Here's how the part is built. I have some questions about the finished solid (model axes, mm). A direction names the side the tool comes from. Coordinates: 2 decimals unless noted, no trailing zeros. Order: outer loops, then holes, each group sorted by start corner. A loop starts at its lowest first (then second) coordinate and runs counter-clockwise, first axis right, second up. Notation, with made-up numbers: (76.25, 55) - (94.25, 55) arc R31 cw to (94.25, 89) - close; hole circle Ø5 at (-29, 45.25). An arc over 180 degrees is marked (long way). Answer as CSV lines item,"result". Start each with the question number.
Q1. For faces 5 (the face through (-12, 0, -1.5)), 6 (the face through (-12, 0, 1.5)), 7 (the face through (-0.08, -0.62, 8.93)), which set-ups out of +Z, -Z, +X, -X, +Y, -Y let a thin tool reach every point of the face, with its end or its side?
Q2. Thinking about a two-plate mould opening in Z: for faces 1 (the face through (12, 0, 1.5)), 2 (the face through (-5, 1, 8)), 3 (the face through (12, 0, -1.5)), 4 (the face through (13.196, -0.014, -0.065)), which applies, released by +Z, released by -Z, zero draft, split by the parting line, or undercut?
Q3. I need wall thicknesses on line 1 (X direction, y = 0.65, z = 2.5); line 2 (X direction, y = -0.5, z = -3.25); line 3 (Z direction, x = 11.5, y = 0.8). Which ranges of each line are inside material? Lowest first, please.
Q4. Suppose I cut it at C-C (x = -10.25). Please give me the cut outline in (y, z).
Q5. Suppose I cut it at A-A (x = 12.7). Please give me the cut outline in (y, z).
Q6. Suppose I cut it at B-B (y = -0.35). Count the separate pieces of the cut face and the enclosed holes in it, then the cut area to 3 significant figures.
Q7. For pin 1 Ø1 at (x, y) = (-1, 0) entering from -Z; pin 2 Ø8 at (x, z) = (3.5, 3) entering from +Y; pin 3 Ø1 at (x, y) = (-8, -0.5) entering from -Z; pin 4 Ø8 at (x, z) = (-7.5, 1.5) entering from +Y, each with a flat end and sliding along its axis, tell me the tip position at first contact or that it passes through.
from build123d import *

# Parameters (mm, degrees)
SKETCH1_R           = 0.5
BOSS_EXTRUDE1_DEPTH = 1
CUT_EXTRUDE1_START  = -15
CUT_EXTRUDE1_DEPTH  = 30


with BuildPart() as part:
    # Sketch1 → Boss-Extrude1 (new, symmetric)
    # profile 1 of 14: a face of its own
    with BuildSketch(Plane(origin=(0, 0, 0), x_dir=(1, 0, 0), z_dir=(0, 1, 0))):
        with BuildLine():
            Line((-15, -1.5), (-9.886859967, -1.5))
            ThreePointArc((-9.886859967, -1.5), (-10, 0), (-9.886859967, 1.5))
            Line((-9.886859967, 1.5), (-15, 1.5))
            Line((-15, 1.5), (-15, -1.5))
        make_face()
        with Locations(Location((-12.7, 0, 0), (0, 0, 270))):
            Circle(SKETCH1_R, mode=Mode.SUBTRACT)
    # profile 2 of 14: a face of its own
    with BuildSketch(Plane(origin=(0, 0, 0), x_dir=(1, 0, 0), z_dir=(0, 1, 0))):
        with BuildLine():
            ThreePointArc((-9.886859967, 1.5), (-10, 0), (-9.886859967, -1.5))
            Line((-9.886859967, -1.5), (-8.874119675, -1.5))
            ThreePointArc((-8.874119675, -1.5), (-9, 0), (-8.874119675, 1.5))
            Line((-8.874119675, 1.5), (-9.886859967, 1.5))
        make_face()
    # profile 3 of 14: a face of its own
    with BuildSketch(Plane(origin=(0, 0, 0), x_dir=(1, 0, 0), z_dir=(0, 1, 0))):
        with BuildLine():
            Line((8.874119675, -1.5), (9.886859967, -1.5))
            ThreePointArc((9.886859967, -1.5), (9.971674876, -0.752130419), (10, 0))
            ThreePointArc((10, 0), (9.971674876, 0.752130419), (9.886859967, 1.5))
            Line((9.886859967, 1.5), (8.874119675, 1.5))
            ThreePointArc((8.874119675, 1.5), (8.968474705, 0.752636343), (9, 0))
            ThreePointArc((9, 0), (8.968474705, -0.752636343), (8.874119675, -1.5))
        make_face()
    # profile 4 of 14: a face of its own
    with BuildSketch(Plane(origin=(0, 0, 0), x_dir=(1, 0, 0), z_dir=(0, 1, 0))):
        with BuildLine():
            ThreePointArc((-9.886859967, -1.5), (-6.519202405, -7.582875444), (0, -10))
            Line((0, -10), (0, -9))
            ThreePointArc((0, -9), (-5.809475019, -6.873863542), (-8.874119675, -1.5))
            Line((-8.874119675, -1.5), (-9.886859967, -1.5))
        make_face()
    # profile 5 of 14: a face of its own
    with BuildSketch(Plane(origin=(0, 0, 0), x_dir=(1, 0, 0), z_dir=(0, 1, 0))):
        with BuildLine():
            Line((0, -9), (0, -10))
            ThreePointArc((0, -10), (6.519202405, -7.582875444), (9.886859967, -1.5))
            Line((9.886859967, -1.5), (8.874119675, -1.5))
            ThreePointArc((8.874119675, -1.5), (5.809475019, -6.873863542), (0, -9))
        make_face()
    # profile 6 of 14: a face of its own
    with BuildSketch(Plane(origin=(0, 0, 0), x_dir=(1, 0, 0), z_dir=(0, 1, 0))):
        with BuildLine():
            ThreePointArc((0, 10), (-6.519202405, 7.582875444), (-9.886859967, 1.5))
            Line((-9.886859967, 1.5), (-8.874119675, 1.5))
            ThreePointArc((-8.874119675, 1.5), (-5.809475019, 6.873863542), (0, 9))
            Line((0, 9), (0, 10))
        make_face()
    # profile 7 of 14: a face of its own
    with BuildSketch(Plane(origin=(0, 0, 0), x_dir=(1, 0, 0), z_dir=(0, 1, 0))):
        with BuildLine():
            ThreePointArc((9.886859967, 1.5), (6.519202405, 7.582875444), (0, 10))
            Line((0, 10), (0, 9))
            ThreePointArc((0, 9), (5.809475019, 6.873863542), (8.874119675, 1.5))
            Line((8.874119675, 1.5), (9.886859967, 1.5))
        make_face()
    # profile 8 of 14: a face of its own
    with BuildSketch(Plane(origin=(0, 0, 0), x_dir=(1, 0, 0), z_dir=(0, 1, 0))):
        with BuildLine():
            ThreePointArc((-9.886859967, -1.5), (-6.519202405, -7.582875444), (0, -10))
            Line((0, -10), (0, -9))
            ThreePointArc((0, -9), (-5.809475019, -6.873863542), (-8.874119675, -1.5))
            Line((-8.874119675, -1.5), (-9.886859967, -1.5))
        make_face()
    # profile 9 of 14: a face of its own
    with BuildSketch(Plane(origin=(0, 0, 0), x_dir=(1, 0, 0), z_dir=(0, 1, 0))):
        with BuildLine():
            Line((0, -9), (0, -10))
            ThreePointArc((0, -10), (6.519202405, -7.582875444), (9.886859967, -1.5))
            Line((9.886859967, -1.5), (8.874119675, -1.5))
            ThreePointArc((8.874119675, -1.5), (5.809475019, -6.873863542), (0, -9))
        make_face()
    # profile 10 of 14: a face of its own
    with BuildSketch(Plane(origin=(0, 0, 0), x_dir=(1, 0, 0), z_dir=(0, 1, 0))):
        with BuildLine():
            ThreePointArc((0, 10), (-6.519202405, 7.582875444), (-9.886859967, 1.5))
            Line((-9.886859967, 1.5), (-8.874119675, 1.5))
            ThreePointArc((-8.874119675, 1.5), (-5.809475019, 6.873863542), (0, 9))
            Line((0, 9), (0, 10))
        make_face()
    # profile 11 of 14: a face of its own
    with BuildSketch(Plane(origin=(0, 0, 0), x_dir=(1, 0, 0), z_dir=(0, 1, 0))):
        with BuildLine():
            ThreePointArc((9.886859967, 1.5), (6.519202405, 7.582875444), (0, 10))
            Line((0, 10), (0, 9))
            ThreePointArc((0, 9), (5.809475019, 6.873863542), (8.874119675, 1.5))
            Line((8.874119675, 1.5), (9.886859967, 1.5))
        make_face()
    # profile 12 of 14: a face of its own
    with BuildSketch(Plane(origin=(0, 0, 0), x_dir=(1, 0, 0), z_dir=(0, 1, 0))):
        with BuildLine():
            ThreePointArc((10, 0), (9.971674876, -0.752130419), (9.886859967, -1.5))
            Line((9.886859967, -1.5), (15, -1.5))
            Line((15, -1.5), (15, 1.5))
            Line((15, 1.5), (9.886859967, 1.5))
            ThreePointArc((9.886859967, 1.5), (9.971674876, 0.752130419), (10, 0))
        make_face()
        with Locations(Location((12.7, 0, 0), (0, 0, 270))):
            Circle(SKETCH1_R, mode=Mode.SUBTRACT)
    # profile 13 of 14: a face of its own
    with BuildSketch(Plane(origin=(0, 0, 0), x_dir=(1, 0, 0), z_dir=(0, 1, 0))):
        with BuildLine():
            ThreePointArc((-9.886859967, 1.5), (-10, 0), (-9.886859967, -1.5))
            Line((-9.886859967, -1.5), (-8.874119675, -1.5))
            ThreePointArc((-8.874119675, -1.5), (-9, 0), (-8.874119675, 1.5))
            Line((-8.874119675, 1.5), (-9.886859967, 1.5))
        make_face()
    # profile 14 of 14: a face of its own
    with BuildSketch(Plane(origin=(0, 0, 0), x_dir=(1, 0, 0), z_dir=(0, 1, 0))):
        with BuildLine():
            Line((8.874119675, -1.5), (9.886859967, -1.5))
            ThreePointArc((9.886859967, -1.5), (9.971674876, -0.752130419), (10, 0))
            ThreePointArc((10, 0), (9.971674876, 0.752130419), (9.886859967, 1.5))
            Line((9.886859967, 1.5), (8.874119675, 1.5))
            ThreePointArc((8.874119675, 1.5), (8.968474705, 0.752636343), (9, 0))
            ThreePointArc((9, 0), (8.968474705, -0.752636343), (8.874119675, -1.5))
        make_face()
    extrude(amount=BOSS_EXTRUDE1_DEPTH, both=True)

    # Sketch5 → Revolve1 (revolve)
    with BuildSketch(Plane.XY, mode=Mode.PRIVATE) as revolve1_sk:
        with BuildLine():
            Line((-9, 1.256849708), (-9.256849708, 1))
            Line((-9.256849708, 1), (-9.256849708, -1))
            Line((-9.256849708, -1), (-8, -1))
            Line((-8, -1), (-6, -1))
            add(Edge.make_bspline(
                [(-9, 1.256849708), (-7.866217648, -0.858961069), (-6, -1)],
                knots=[0, 0, 0, 0.981692631, 0.981692631, 0.981692631], degree=2))
        make_face()
    revolve(revolve1_sk.sketch.rotate(Axis((0, -1000, 0), (0, 1, 0)), 180), axis=Axis((0, -1000, 0), (0, 1, 0)))

    # Sketch6 → Cut-Extrude1 (cut)
    with BuildSketch(Plane(origin=(0, 0, 0), x_dir=(0, 0, -1), z_dir=(1, 0, 0)).offset(CUT_EXTRUDE1_START)):
        Polygon((10, 0), (10, -1), (8.267949192, -1), align=None)
        Polygon((-10, 0), (-10, -1), (-8.267949192, -1), align=None)
    extrude(amount=CUT_EXTRUDE1_DEPTH, mode=Mode.SUBTRACT)


solid = part.part
Here are the results:
1,face 5,"-Z, -X, +Y, -Y"
1,face 6,"+Z, -X, +Y, -Y"
1,face 7,"+Z, +X, -X, -Y"
2,face 1,"released by +Z"
2,face 2,"zero draft"
2,face 3,"released by -Z"
2,face 4,"undercut"
3,line 1,"x = -9.68 to -8.26, 8.26 to 9.68"
3,line 2,"x = -9.46 to -6.75, 6.75 to 9.46"
3,line 3,"z = -1.5 to 1.5"
4,outline,"(-1, -1.5) - (1, -1.5) - (1, 1.5) - (-1, 1.5) - close"
5,outline,"(-1, -1.5) - (1, -1.5) - (1, -0.5) - (-1, -0.5) - close; (-1, 0.5) - (1, 0.5) - (1, 1.5) - (-1, 1.5) - close"
6,separate pieces,"1"
6,enclosed holes,"3"
6,area,"151 mm²"
7,pin 1,"stops at z = -9.99"
7,pin 2,"stops at y = 0.62"
7,pin 3,"stops at z = -6.61"
7,pin 4,"stops at y = 1.26"
